Part model, mm, in its own coordinate system. Face numbers are marked on the shaded views. A direction names the side the tool comes from. Round coordinates to 2 decimals unless told otherwise and drop trailing zeros. Write each loop counter-clockwise with the first axis right and the second up, starting at its lowest first coordinate (ties: lowest second). Pieces come first, ordered by that corner, then holes. Notation, with made-up numbers: M 48.5,52 L 86.5,52 A28 ccw 86.5,80 Z; hole C 6.25,-37.5 d9. An arc over 180 degrees is marked long. Use a Markdown table: item, result. Add a question column.
1) Slice it at B-B on x = 0. Write the cut outline in (y, z).
2) Slice it at D-D on y = 0. Write the cut outline in (x, z).
3) Two-plate mould, pull along Y, no slides. Class the marked faces 5, 6 and 7: released by +Y, released by -Y, zero draft, split by the parting line, or undercut.
4) Drop flat-ended pins along their axis: P1, Ø1.5, axis at y = -48.5, z = 36, coming from the +X side; P2, Ø6.5, axis at x = 24.5, z = -5, coming from the +Y side; P3, Ø18, axis at y = 25, z = -25, coming from the +X side. Give the stop position or say it passes through.
5) Which spindle directions (+Z, -Z, +X, -X, +Y, -Y) get a long thin tool onto all of the face, cutting with end or side? Do the marked faces 1, 2, 3 and 4. Say none if no direction does.
6) Wall check: probe 1 along Z at (x, y) = (0, -47.3); probe 2 along Z at (x, y) = (-47.1, 25); probe 3 along X at (y, z) = (-25, -49). Give the ranges that are in metal, low to high.
7) Slice it at C-C on z = 0. Write the cut outline in (x, y).
```python
from build123d import *

# Parameters (mm, degrees)
F0_W      = 100
F0_H      = 100
F1_DEPTH  = 50
F2_R      = 17.5
F3_DEPTH  = 4
F4_R      = 15
F5_DEPTH  = 4
F6_R      = 13
F7_DEPTH  = 4
F8_R      = 14.5
F9_DEPTH  = 4
F10_R     = 12.5
F11_DEPTH = 4
F12_R     = 11
F13_DEPTH = 4
F14_R     = 3
F15_W     = 6
F15_H     = 6
F16_DEPTH = 5


with BuildPart() as f1:
    # F0 (on Top) → F1 (new body, symmetric)
    with BuildSketch(Plane.XY):
        Rectangle(F0_W, F0_H)
    extrude(amount=F1_DEPTH, both=True)

    # F2 (on face) → F3 (cut)
    with BuildSketch(Plane.XZ.offset(50)):
        Circle(F2_R)
    extrude(amount=-F3_DEPTH, mode=Mode.SUBTRACT)

    # F4 (on face) → F5 (cut)
    with BuildSketch(Plane.YZ.offset(50)):
        with Locations((-25, 25)):
            Circle(F4_R)
        with Locations((25, -25)):
            Circle(F4_R)
    extrude(amount=-F5_DEPTH, mode=Mode.SUBTRACT)

    # F6 (on face) → F7 (cut)
    with BuildSketch(Plane.XY.offset(50)):
        with Locations((-25, 25)):
            Circle(F6_R)
        with BuildLine():
            Line((-13, 0), (13, 0))
            ThreePointArc((13, 0), (0, 13), (-13, 0))
        make_face()
        with BuildLine():
            ThreePointArc((-13, 0), (0, -13), (13, 0))
            Line((13, 0), (-13, 0))
        make_face()
        with Locations((25, -25)):
            Circle(F6_R)
    extrude(amount=-F7_DEPTH, mode=Mode.SUBTRACT)

    # F8 (on face) → F9 (cut)
    with BuildSketch(Plane(origin=(0, 0, -50), x_dir=(1, 0, 0), z_dir=(0, 0, -1))):
        with Locations((-25, 25)):
            Circle(F8_R)
        with Locations((25, 25)):
            Circle(F8_R)
        with Locations((-25, -25)):
            Circle(F8_R)
        with Locations((25, -25)):
            Circle(F8_R)
    extrude(amount=-F9_DEPTH, mode=Mode.SUBTRACT)

    # F10 (on face) → F11 (cut)
    with BuildSketch(Plane(origin=(-50, 0, 0), x_dir=(0, -1, 0), z_dir=(-1, 0, 0))):
        Circle(F10_R)
        with Locations((25, 25)):
            Circle(F10_R)
        with Locations((-25, 25)):
            Circle(F10_R)
        with Locations((-25, -25)):
            Circle(F10_R)
        with Locations((25, -25)):
            Circle(F10_R)
    extrude(amount=-F11_DEPTH, mode=Mode.SUBTRACT)

    # F12 (on face) → F13 (cut)
    with BuildSketch(Plane(origin=(0, 50, 0), x_dir=(-1, 0, 0), z_dir=(0, 1, 0))):
        with Locations((-25, 0)):
            Circle(F12_R)
        with Locations((-25, 25)):
            Circle(F12_R)
        with Locations((-25, -25)):
            Circle(F12_R)
        with Locations((25, -25)):
            Circle(F12_R)
        with Locations((25, 0)):
            Circle(F12_R)
        with Locations((25, 25)):
            Circle(F12_R)
    extrude(amount=-F13_DEPTH, mode=Mode.SUBTRACT)

    # F14
    f14_edges = [f1.edges().sort_by_distance(p)[0] for p in [
        (50, 0, 50),
        (0, 50, 50),
        (-50, 0, 50),
        (0, -50, 50),
        (-50, -50, 0),
        (0, -50, -50),
        (50, -50, 0),
        (50, 0, -50),
        (0, 50, -50),
        (50, 50, 0),
        (-50, 50, 0),
        (-50, 0, -50),
    ]]
    fillet(f14_edges, radius=F14_R)

    # F15 (on face) → F16 (cut)
    with BuildSketch(Plane.XZ.offset(50)):
        with Locations((-36.2572609186, 37.3459062278)):
            Rectangle(F15_W, F15_H)
        with Locations((-24.2572609186, 37.3459062278)):
            Rectangle(F15_W, F15_H)
        with Locations((-12.2572609186, 37.3459062278)):
            Rectangle(F15_W, F15_H)
        with Locations((-0.2572609186, 37.3459062278)):
            Rectangle(F15_W, F15_H)
        with Locations((11.7427390814, 37.3459062278)):
            Rectangle(F15_W, F15_H)
        with Locations((23.7427390814, 37.3459062278)):
            Rectangle(F15_W, F15_H)
        with Locations((35.7427390814, 37.3459062278)):
            Rectangle(F15_W, F15_H)
    extrude(amount=-F16_DEPTH, mode=Mode.SUBTRACT)


solid = f1.part
```
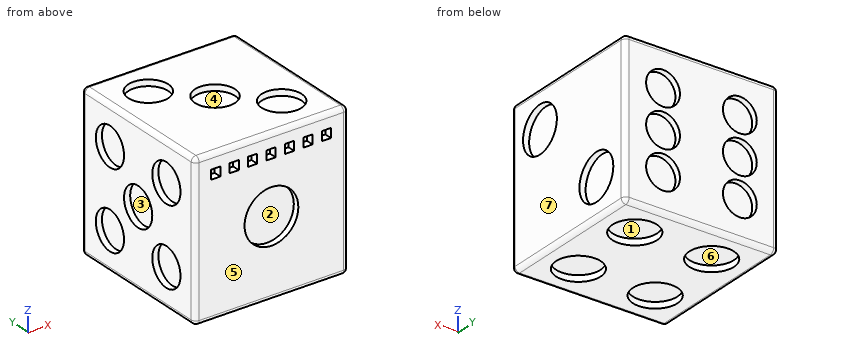
Entries:
| question | item | result |
|---|---|---|
| 1 | outline | M -50,-47 A3 ccw -47,-50 L 47,-50 A3 ccw 50,-47 L 50,47 A3 ccw 47,50 L 13,50 L 13,46 L -13,46 L -13,50 L -47,50 A3 ccw -50,47 L -50,40.35 L -45,40.35 L -45,34.35 L -50,34.35 L -50,17.5 L -46,17.5 L -46,-17.5 L -50,-17.5 Z |
| 2 | outline | M -50,-47 A3 ccw -47,-50 L 47,-50 A3 ccw 50,-47 L 50,47 A3 ccw 47,50 L 13,50 L 13,46 L -13,46 L -13,50 L -47,50 A3 ccw -50,47 L -50,12.5 L -46,12.5 L -46,-12.5 L -50,-12.5 Z |
| 3 | face 5 | released by -Y |
| 3 | face 6 | undercut |
| 3 | face 7 | zero draft |
| 4 | P1 | stops at x = 49.9 |
| 4 | P2 | stops at y = 46 |
| 4 | P3 | stops at x = 46 |
| 5 | face 1 | -Z |
| 5 | face 2 | -Y |
| 5 | face 3 | -X |
| 5 | face 4 | +Z |
| 6 | probe 1 | z = -49.98 to -17.5, 17.5 to 34.35, 40.35 to 49.98 |
| 6 | probe 2 | z = -50 to -37.5, -12.5 to 12.5, 37.5 to 50 |
| 6 | probe 3 | x = -49.24 to -39.5, -10.5 to 10.5, 39.5 to 49.24 |
| 7 | outline | M -50,-47 A3 ccw -47,-50 L -17.5,-50 L -17.5,-46 L 17.5,-46 L 17.5,-50 L 47,-50 A3 ccw 50,-47 L 50,47 A3 ccw 47,50 L 36,50 L 36,46 L 14,46 L 14,50 L -14,50 L -14,46 L -36,46 L -36,50 L -47,50 A3 ccw -50,47 L -50,12.5 L -46,12.5 L -46,-12.5 L -50,-12.5 Z |
